Here's the drawing with two shaded views (mm, measured from the low corner). I have some questions. A direction names the side the tool comes from. Round coordinates to 2 decimals unless told otherwise and drop trailing zeros. Loops run counter-clockwise (first coordinate to the right, second up) from the corner with the lowest first, then second, coordinate; pieces in that order, holes last.
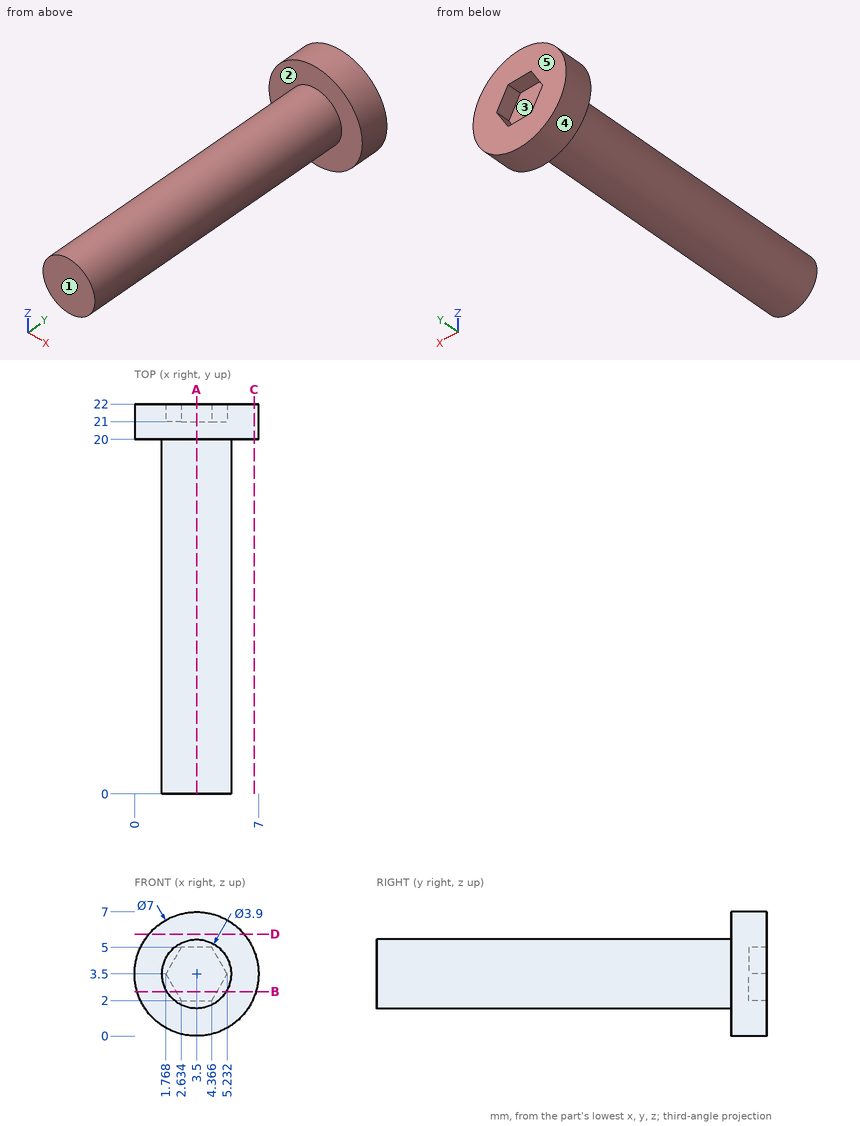
Item 1: If we section it at B-B, the plane z = 2.5: Please give me the cut outline in (x, y), then the cut area to 3 significant figures.
Results list:
outline: (0.15, 20) - (1.83, 20) - (1.83, 0) - (5.17, 0) - (5.17, 20) - (6.85, 20) - (6.85, 22) - (4.65, 22) - (4.65, 21) - (2.35, 21) - (2.35, 22) - (0.15, 22) - close
area: 78.1 mm2
Item 2: For the marked faces 1 and 2, which set-ups out of +Z, -Z, +X, -X, +Y, -Y let a thin tool reach every point of the face, with its end or its side?
Results list:
face 1: +Z, -Z, +X, -X, -Y
face 2: -Y
Item 3: Will this pin go through, and if not, where does the flat tip stop? pin 1 (4 mm diameter, centred on x = 6, y = 16.5, fed in from -Z) (3 decimals).
Results list:
pin 1: stops at z = 1.615
Item 4: If we section it at C-C, the plane x = 6.75: Please give me the cut outline in (y, z).
Results list:
outline: (20, 2.2) - (22, 2.2) - (22, 4.8) - (20, 4.8) - close
Item 5: We'd pull the mould along Z, two halves only. Please class the marked faces 3, 4 and 5: released by +Z, released by -Z, zero draft, split by the parting line, or undercut.
Results list:
face 3: undercut
face 4: split by the parting line
face 5: zero draft
Item 6: If I drill on line 1 along Z through (x, y) = (3.5, 18.25); line 2 along Y through (x, z) = (0.5, 3); line 3 along Y through (x, z) = (5, 3.25), over which ranges is the centre line in solid material (lowest first)?
Results list:
line 1: z = 1.55 to 5.45
line 2: y = 20 to 22
line 3: y = 0 to 21
Item 7: If we section it at D-D, the plane z = 5.75: Please give me the cut outline in (x, y).
Results list:
outline: (0.82, 20) - (6.18, 20) - (6.18, 22) - (0.82, 22) - close
Item 8: If we section it at A-A, the plane x = 3.5: Please give me the cut outline in (y, z), then the cut area to 3 significant figures.
Results list:
outline: (0, 1.55) - (20, 1.55) - (20, 0) - (22, 0) - (22, 2) - (21, 2) - (21, 5) - (22, 5) - (22, 7) - (20, 7) - (20, 5.45) - (0, 5.45) - close
area: 89.0 mm2
